Geometry: final body of the model. Coordinates: model frame, mm. Face numbers are marked on the shaded views. A direction names the side the tool comes from. Round coordinates to 2 decimals unless told otherwise and drop trailing zeros. Loops run counter-clockwise (first coordinate to the right, second up) from the corner with the lowest first, then second, coordinate; pieces in that order, holes last. Notation, with made-up numbers: (-27.5, 89.25) - (-1.5, 89.25) arc R23 cw to (-1.5, 104.25) - close; hole circle Ø9 at (20.5, 87). An arc over 180 degrees is marked (long way). Answer as CSV lines item,"result".
from build123d import *

# Parameters (mm, degrees)
SKETCH1_R               = 20
BOSS_EXTRUDE1_DEPTH     = 52
CUT_EXTRUDE1_DEPTH      = 60.194594348
CUT_EXTRUDE1_DEPTH_BACK = 60.194594348
SKETCH2_R               = 10
BOSS_EXTRUDE8_DEPTH     = 12
SKETCH7_R               = 10
BOSS_EXTRUDE9_DEPTH     = 30
CUT_EXTRUDE2_DEPTH      = 115.47270417
CUT_EXTRUDE2_DEPTH_BACK = 24
SKETCH9_R               = 6
FILLET1_R               = 6
CUT_EXTRUDE3_DEPTH      = 124.304501177
CUT_EXTRUDE3_DEPTH_BACK = 124.304501177
SKETCH11_W              = 42.326213612
SKETCH11_H              = 24


with BuildPart() as part:
    # Sketch1 → Boss-Extrude1 (new body)
    with BuildSketch(Plane(origin=(0, 0, 0), x_dir=(1, 0, 0), z_dir=(0, 1, 0))):
        with Locations(Location((0, 0, 0), (0, 0, 90))):
            Circle(SKETCH1_R)
    extrude(amount=BOSS_EXTRUDE1_DEPTH)

    # Sketch2 → Cut-Extrude1 (cut, two sides: drawn at the far end of the back side and taken through both)
    with BuildSketch(Plane(origin=(0, 52, 0), x_dir=(1, 0, 0), z_dir=(0, 1, 0)).offset(-CUT_EXTRUDE1_DEPTH_BACK)):
        with Locations(Location((0, 0, 0), (0, 0, 270))):
            Circle(SKETCH2_R)
    extrude(amount=CUT_EXTRUDE1_DEPTH + CUT_EXTRUDE1_DEPTH_BACK, mode=Mode.SUBTRACT)

    # Sketch5 → Boss-Extrude8 (add, symmetric)
    with BuildSketch(Plane.XY):
        with BuildLine():
            Line((26, 0), (16, 0))
            Line((16, 0), (16, 14))
            Line((16, 14), (26, 14))
            ThreePointArc((26, 14), (38, 26), (26, 38))
            Line((26, 38), (16, 38))
            Line((16, 38), (16, 52))
            Line((16, 52), (26, 52))
            ThreePointArc((26, 52), (39.490737563, 48.226110771), (49.065125189, 38))
            Line((49.065125189, 38), (80, 38))
            Line((80, 38), (80, 14))
            Line((80, 14), (49.065125189, 14))
            ThreePointArc((49.065125189, 14), (39.490737563, 3.773889229), (26, 0))
        make_face()
    extrude(amount=BOSS_EXTRUDE8_DEPTH, both=True)

    # Sketch7 → Boss-Extrude9 (add)
    with BuildSketch(Plane(origin=(80, 0, 0), x_dir=(0, 0, -1), z_dir=(1, 0, 0))):
        with Locations((0, 26)):
            Circle(SKETCH7_R)
    extrude(amount=BOSS_EXTRUDE9_DEPTH)

    # Sketch9 → Cut-Extrude2 (cut, two sides: drawn at the far end of the back side and taken through both)
    with BuildSketch(Plane(origin=(80, 0, 0), x_dir=(0, 0, -1), z_dir=(1, 0, 0)).offset(-CUT_EXTRUDE2_DEPTH_BACK)):
        with Locations((-12, 38)):
            Circle(SKETCH9_R)
        with Locations((12, 38)):
            Circle(SKETCH9_R)
        with Locations((12, 14)):
            Circle(SKETCH9_R)
        with Locations((-12, 14)):
            Circle(SKETCH9_R)
    extrude(amount=CUT_EXTRUDE2_DEPTH + CUT_EXTRUDE2_DEPTH_BACK, mode=Mode.SUBTRACT)

    # Fillet1
    fillet1_edges = [part.edges().sort_by_distance(p)[0] for p in [
        (56, 18.242640687, -7.757359313),
        (56, 18.242640687, 7.757359313),
        (56, 33.757359313, -7.757359313),
        (56, 33.757359313, 7.757359313),
    ]]
    fillet(fillet1_edges, radius=FILLET1_R - 0.0001)  # a hair under: the kernel refuses the full size

    # Sketch11 → Cut-Extrude3 (cut, two sides: drawn at the far end of the back side and taken through both)
    with BuildSketch(Plane.XY.offset(-CUT_EXTRUDE3_DEPTH_BACK)):
        with Locations((0, 26)):
            Rectangle(SKETCH11_W, SKETCH11_H)
    extrude(amount=CUT_EXTRUDE3_DEPTH + CUT_EXTRUDE3_DEPTH_BACK, mode=Mode.SUBTRACT)


solid = part.part
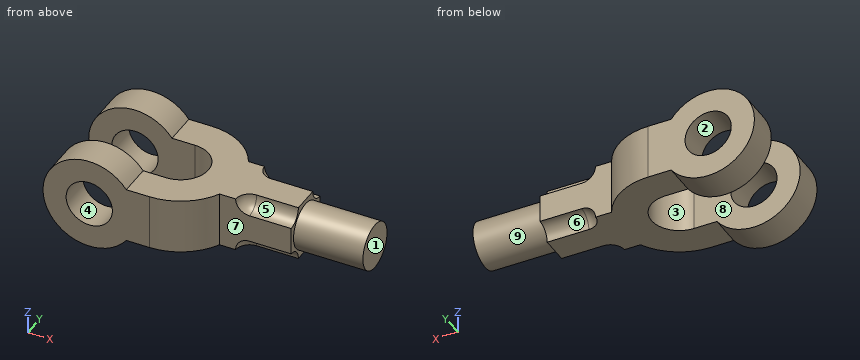
(1) Section A-A (z = 0). Output: boundary loops of the cut face in (x, y).
Findings below:
outline,"(-20, 0) - (-10, 0) - (-10, 14) - (-20, 14) - close; (-20, 38) - (-10, 38) - (-10, 52) - (-20, 52) - close; (10, 0) - (26, 0) arc R26 ccw to (49.07, 14) - (80, 14) - (80, 16) - (110, 16) - (110, 36) - (80, 36) - (80, 38) - (49.07, 38) arc R26 ccw to (26, 52) - (10, 52) - (10, 38) - (26, 38) arc R12 cw to (26, 14) - (10, 14) - close"
(2) Draft query along X for the marked faces 1, 2, 3 and 4. Return one class per face: pulls with the +X half, pulls with the -X half, needs draft (parallel to the pull), parting line crosses it, or undercut.
Findings below:
face 1,"pulls with the +X half"
face 2,"undercut"
face 3,"pulls with the -X half"
face 4,"undercut"
(3) Pin query (flat end, axial travel): P1, Ø23, axis at x = 0, z = 0, coming from the -Y side; P2, Ø18, axis at x = 0, z = 0, coming from the +Y side; P3, Ø1, axis at y = 18.5, z = -8, coming from the -X side; P4, Ø19, axis at x = 62.5, z = 5.5, coming from the +Y side. Return the tip coordinate at first contact, or that it passes through.
Findings below:
P1,"y = 0"
P2,"through"
P3,"x = 34.94"
P4,"y = 38"
(4) Material intervals for line 1 along Z through (x, y) = (-0.5, 49.5); line 2 along Y through (x, z) = (-4.5, -13.5); line 3 along Y through (x, z) = (66.5, 2.5), sorted ascending.
Findings below:
line 1,"-19.99 to -9.99, 9.99 to 19.99"
line 2,"0 to 14, 38 to 52"
line 3,"14 to 38"
(5) Access query for the marked faces 5, 6, 7, 8 and 9. Directions: +Z, -Z, +X, -X, +Y, -Y. A direction counts if a zero-diameter tool reaches every point of the face in a straight line with its end or side. Return the directions, or none.
Findings below:
face 5,"+Z, +X, -Y"
face 6,"-Z, +X, +Y"
face 7,"+Z, -Z, +X, -Y"
face 8,"+Z, -Z, -X"
face 9,"+X"
(6) Section B-B (x = 0). Output: boundary loops of the cut face in (y, z), and give its area (3 significant figures).
Findings below:
outline,"(0, -20) - (14, -20) - (14, -10) - (0, -10) - close; (0, 10) - (14, 10) - (14, 20) - (0, 20) - close; (38, -20) - (52, -20) - (52, -10) - (38, -10) - close; (38, 10) - (52, 10) - (52, 20) - (38, 20) - close"
area,"560 mm2"
(7) Section C-C (x = 23). Output: boundary loops of the cut face in (y, z), and give its area (3 significant figures).
Findings below:
outline,"(0, -12) - (14, -12) - (14, 12) - (0, 12) - close; (38, -12) - (52, -12) - (52, 12) - (38, 12) - close"
area,"672 mm2"
(8) Section D-D (z = 15.5). Output: boundary loops of the cut face in (x, y), and give its area (3 significant figures).
Findings below:
outline,"(-12.64, 0) - (12.64, 0) - (12.64, 14) - (-12.64, 14) - close; (-12.64, 38) - (12.64, 38) - (12.64, 52) - (-12.64, 52) - close"
area,"708 mm2"
